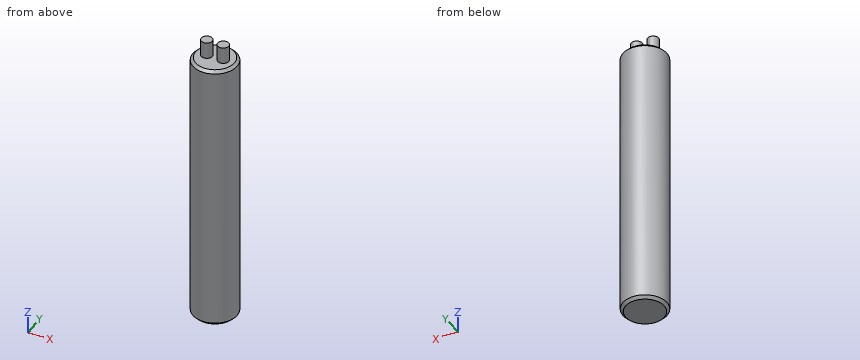
```python
from build123d import *

# Parameters (mm, degrees)
F0_R     = 4
F1_DEPTH = 50
F2_SIZE  = 0.5
F3_R     = 1
F4_DEPTH = 3


with BuildPart() as f1:
    # F0 (on Top) → F1 (new body)
    with BuildSketch(Plane.XY):
        Circle(F0_R)
    extrude(amount=F1_DEPTH)

    # F2
    f2_edges = [f1.edges().sort_by_distance(p)[0] for p in [
        (-4, 0, 50),
        (-4, 0, 0),
    ]]
    chamfer(f2_edges, length=F2_SIZE)

    # F3 (on face) → F4 (join)
    with BuildSketch(Plane.XY.offset(50)):
        with Locations((1.5, 0)):
            Circle(F3_R)
        with Locations((-1.5, 0)):
            Circle(F3_R)
    extrude(amount=F4_DEPTH)


solid = f1.part
```
Model file for the job. Use its own axes, mm. Give positions to 0.01 mm unless a question says otherwise; leave off trailing zeros. Loops run counter-clockwise (first coordinate to the right, second up) from the corner with the lowest first, then second, coordinate; pieces in that order, holes last. Notation, with made-up numbers: (17, 20) - (29, 20) arc R18 ccw to (29, 52) - close; hole circle Ø8 at (28.5, 36). An arc over 180 degrees is marked (long way). One line per item, written item: value. Start each with the question number.
1. Probe L1, parallel to Z at x = -3, y = -1; L2, parallel to X at y = -1.25, z = 7; L3, parallel to Y at x = 0.25, z = 12. List the from-to ranges inside material, lowest first. Write a range as from..to.
2. Slice it at A-A (x = 0). List the corners of the cut face in (y, z).
3. Slice it at B-B (y = 0). List the corners of the cut face in (x, z), plus the area to 4 significant figures.
4. Slice it at C-C (z = 45). List the corners of the cut face in (x, y).
Solution:
1. L1: z = 0..50
1. L2: x = -3.8..3.8
1. L3: y = -3.99..3.99
2. outline: (-4, 0.5) - (-3.5, 0) - (3.5, 0) - (4, 0.5) - (4, 49.5) - (3.5, 50) - (-3.5, 50) - (-4, 49.5) - close
3. outline: (-4, 0.5) - (-3.5, 0) - (3.5, 0) - (4, 0.5) - (4, 49.5) - (3.5, 50) - (2.5, 50) - (2.5, 53) - (0.5, 53) - (0.5, 50) - (-0.5, 50) - (-0.5, 53) - (-2.5, 53) - (-2.5, 50) - (-3.5, 50) - (-4, 49.5) - close
3. area: 411.5 mm^2
4. outline: circle Ø8 at (0, 0)
